Here's how the part is built. I have some questions about the finished solid (model axes, mm). Face numbers are marked on the shaded views. A direction names the side the tool comes from. Give positions to 0.01 mm unless a question says otherwise; leave off trailing zeros. Loops run counter-clockwise (first coordinate to the right, second up) from the corner with the lowest first, then second, coordinate; pieces in that order, holes last.
Q1. If we section it at C-C (x = -18.5): Please give me the cut outline in (y, z).
Q2. We'd pull the mould along X, two halves only. Please class the marked faces 1, 2 and 3: +X half, -X half, draft (parallel to the pull), parting line (faces both ways), or undercut.
Q3. I need wall thicknesses on line 1 (Y direction, x = -70, z = -1); line 2 (X direction, y = 108, z = -4); line 3 (Y direction, x = 38, z = -4.75). Which ranges of each line are inside material? Lowest first, please.
Q4. If we section it at B-B (z = 3): Please give me the cut outline in (x, y), plus the area to 3 significant figures.
Q5. Will these pins go through, and if not, where does the flat tip stop? P1, Ø10, axis at x = 18.5, z = 3, coming from the +Y side; P2, Ø1.4, axis at y = 88.5, z = -6.5, coming from the +X side; P3, Ø10.5, axis at x = -70, y = 7.5, coming from the -Z side; P4, Ø1.4, axis at y = 77.5, z = -7, coming from the -X side.
Q6. If we section it at A-A (y = 123.5): Please give me the cut outline in (x, z).
Q7. For the marked faces 4, 5 and 6, which set-ups out of +Z, -Z, +X, -X, +Y, -Y let a thin tool reach every point of the face, with its end or its side?
from build123d import *

# Parameters (mm, degrees)
SKETCH1_R           = 4.05
BOSS_EXTRUDE1_DEPTH = 10
CUT_EXTRUDE1_DEPTH  = 135


with BuildPart() as part:
    # Sketch1 → Boss-Extrude1 (new, symmetric)
    with BuildSketch(Plane.XY):
        with BuildLine():
            Line((-77.5, 0), (77.5, 0))
            Line((77.5, 0), (77.5, 7.5))
            ThreePointArc((77.5, 7.5), (75.303300859, 12.803300859), (70, 15))
            Line((70, 15), (50, 15))
            Line((50, 15), (50, 145))
            Line((50, 145), (-50, 145))
            Line((-50, 145), (-50, 15))
            Line((-50, 15), (-70, 15))
            ThreePointArc((-70, 15), (-75.303300859, 12.803300859), (-77.5, 7.5))
            Line((-77.5, 7.5), (-77.5, 0))
        make_face()
        with Locations((-70, 7.5)):
            Circle(SKETCH1_R, mode=Mode.SUBTRACT)
        with Locations((70, 7.5)):
            Circle(SKETCH1_R, mode=Mode.SUBTRACT)
    extrude(amount=BOSS_EXTRUDE1_DEPTH, both=True)

    # Sketch2 → Cut-Extrude1 (cut)
    with BuildSketch(Plane(origin=(0, 145, 0), x_dir=(1, 0, 0), z_dir=(0, 1, 0))):
        Polygon((-41, -10), (-41, 6.25), (-42.5, 6.25), (-42.5, 7.5), (-41, 7.5), (-41, 10), (41, 10), (41, 7.5), (42.5, 7.5), (42.5, 6.25), (41, 6.25), (41, -10), align=None)
    extrude(amount=-CUT_EXTRUDE1_DEPTH, mode=Mode.SUBTRACT)


solid = part.part
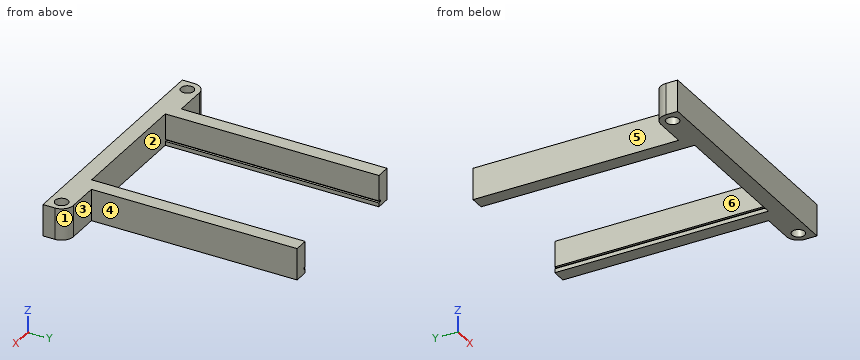
Check sheet entries:
1. outline: (0, -10) - (10, -10) - (10, 10) - (0, 10) - close
2. face 1: +X half
2. face 2: undercut
2. face 3: draft
3. line 1: y = 0 to 3.45, 11.55 to 15
3. line 2: x = -50 to -41, 41 to 50
3. line 3: y = 0 to 10
4. outline: (-77.5, 0) - (77.5, 0) - (77.5, 7.5) arc R7.5 ccw to (70, 15) - (50, 15) - (50, 145) - (41, 145) - (41, 10) - (-41, 10) - (-41, 145) - (-50, 145) - (-50, 15) - (-70, 15) arc R7.5 ccw to (-77.5, 7.5) - close; hole circle Ø8.1 at (-70, 7.5); hole circle Ø8.1 at (70, 7.5)
4. area: 4,130 mm2
5. P1: stops at y = 10
5. P2: stops at x = 50
5. P3: stops at z = -10
5. P4: stops at x = -50
6. outline: (-50, -10) - (-41, -10) - (-41, -7.5) - (-42.5, -7.5) - (-42.5, -6.25) - (-41, -6.25) - (-41, 10) - (-50, 10) - close; (41, -10) - (50, -10) - (50, 10) - (41, 10) - (41, -6.25) - (42.5, -6.25) - (42.5, -7.5) - (41, -7.5) - close
7. face 4: +Z, -Z, +X, +Y
7. face 5: +Z, -Z, -X, +Y
7. face 6: +Z, -Z, +Y
